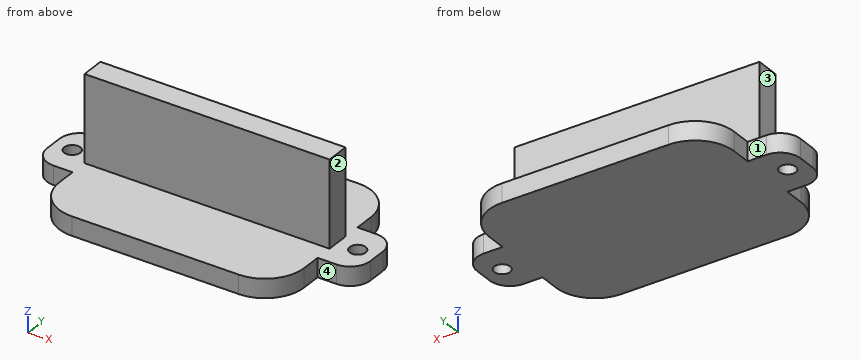
from build123d import *

# Parameters (mm, degrees)
CROQUIS1_R              = 0.85
SALIENTE_EXTRUIR1_DEPTH = 2
CROQUIS2_W              = 26
CROQUIS2_H              = 2.5032448
SALIENTE_EXTRUIR3_DEPTH = 11.15


with BuildPart() as part:
    # Croquis1 → Saliente-Extruir1 (new body)
    # profile 1 of 3: a face of its own
    with BuildSketch(Plane.XY):
        with BuildLine():
            Line((8.85, -9.375), (-8.85, -9.375))
            ThreePointArc((-8.85, -9.375), (-11.784493142, -8.159493142), (-13, -5.225))
            Line((-13, -5.225), (-13, 5.225))
            ThreePointArc((-13, 5.225), (-11.784493142, 8.159493142), (-8.85, 9.375))
            Line((-8.85, 9.375), (8.85, 9.375))
            ThreePointArc((8.85, 9.375), (11.784493142, 8.159493142), (13, 5.225))
            Line((13, 5.225), (13, -5.225))
            ThreePointArc((13, -5.225), (11.784493142, -8.159493142), (8.85, -9.375))
        make_face()
    # profile 2 of 3: a face of its own
    with BuildSketch(Plane.XY):
        with BuildLine():
            Line((-15, -3.125), (-13, -3.125))
            Line((-13, -3.125), (-13, 3.125))
            Line((-13, 3.125), (-15, 3.125))
            ThreePointArc((-15, 3.125), (-16.52027958, 2.49527958), (-17.15, 0.975))
            Line((-17.15, 0.975), (-17.15, -0.975))
            ThreePointArc((-17.15, -0.975), (-16.52027958, -2.49527958), (-15, -3.125))
        make_face()
        with Locations((-15.15, 0)):
            Circle(CROQUIS1_R, mode=Mode.SUBTRACT)
    # profile 3 of 3: a face of its own
    with BuildSketch(Plane.XY):
        with BuildLine():
            Line((13, 3.125), (13, -3.125))
            Line((13, -3.125), (15, -3.125))
            ThreePointArc((15, -3.125), (16.52027958, -2.49527958), (17.15, -0.975))
            Line((17.15, -0.975), (17.15, 0.975))
            ThreePointArc((17.15, 0.975), (16.52027958, 2.49527958), (15, 3.125))
            Line((15, 3.125), (13, 3.125))
        make_face()
        with Locations((15.15, 0)):
            Circle(CROQUIS1_R, mode=Mode.SUBTRACT)
    extrude(amount=SALIENTE_EXTRUIR1_DEPTH)

    # Croquis2 → Saliente-Extruir3 (add)
    with BuildSketch(Plane.XY):
        Rectangle(CROQUIS2_W, CROQUIS2_H)
    extrude(amount=SALIENTE_EXTRUIR3_DEPTH)


solid = part.part
Work out the finished part from the listing and answer in its coordinate system (mm). Face numbers are marked on the shaded views. A direction names the side the tool comes from. Give positions to 0.01 mm unless a question says otherwise; leave off trailing zeros. Order: outer loops, then holes, each group sorted by start corner. A loop starts at its lowest first (then second) coordinate and runs counter-clockwise, first axis right, second up. Notation, with made-up numbers: M 13.5,12.5 L 44.5,12.5 A16 ccw 44.5,42.5 Z; hole C -37.5,52.5 d4. An arc over 180 degrees is marked long. Return JSON: item names as keys, results as strings.
Q1. Each of these flat-tipped pins is pushed along its axis until it touches: pin 1 (1.6 mm diameter, centred on y = -3.5, z = 1, fed in from +X); pin 2 (3 mm diameter, centred on y = -1.5, z = 7.5, fed in from +X); pin 3 (1 mm diameter, centred on x = 15.15, y = 0, fed in from -Z); pin 4 (0.6 mm diameter, centred on y = 4.5, z = 1, fed in from -X). Where does it stop, or does it pass through?
Answer below:
{"pin 1": "stops at x = 16.28", "pin 2": "stops at x = 13", "pin 3": "passes through", "pin 4": "stops at x = -13"}
Q2. Find section B-B, the plane z = 1. Write down the section's boundary in (x, y) (3 decimals), and give its area (3 significant figures).
Answer below:
{"outline": "M -17.15,-0.975 A2.15 ccw -15,-3.125 L -13,-3.125 L -13,-5.225 A4.15 ccw -8.85,-9.375 L 8.85,-9.375 A4.15 ccw 13,-5.225 L 13,-3.125 L 15,-3.125 A2.15 ccw 17.15,-0.975 L 17.15,0.975 A2.15 ccw 15,3.125 L 13,3.125 L 13,5.225 A4.15 ccw 8.85,9.375 L -8.85,9.375 A4.15 ccw -13,5.225 L -13,3.125 L -15,3.125 A2.15 ccw -17.15,0.975 Z; hole C -15.15,0 d1.7; hole C 15.15,0 d1.7", "area": "516 mm^2"}
Q3. Find section A-A, the plane y = 0. Write down the section's boundary in (x, z).
Answer below:
{"outline": "M -17.15,0 L -16,0 L -16,2 L -17.15,2 Z; M -14.3,0 L 14.3,0 L 14.3,2 L 13,2 L 13,11.15 L -13,11.15 L -13,2 L -14.3,2 Z; M 16,0 L 17.15,0 L 17.15,2 L 16,2 Z"}
Q4. Find the intervals of material crossed by line 1 along Y through (x, z) = (-15.15, 0.85); line 2 along Z through (x, y) = (7.5, -4.5); line 3 along Y through (x, z) = (1, 9.75), in increasing order. Write a range as [from, to].
Answer below:
{"line 1": "y = [-3.12, -0.85], [0.85, 3.12]", "line 2": "z = [0, 2]", "line 3": "y = [-1.25, 1.25]"}
Q5. Find section C-C, the plane x = 3. Write down the section's boundary in (y, z) (3 decimals).
Answer below:
{"outline": "M -9.375,0 L 9.375,0 L 9.375,2 L 1.252,2 L 1.252,11.15 L -1.252,11.15 L -1.252,2 L -9.375,2 Z"}
Q6. Find section D-D, the plane z = 8. Write down the section's boundary in (x, y).
Answer below:
{"outline": "M -13,-1.25 L 13,-1.25 L 13,1.25 L -13,1.25 Z"}
Q7. Which of the six approach directions +Z, -Z, +X, -X, +Y, -Y give full straight-line access (tool end or side, diameter ignored) to the marked faces 1, 2, 3 and 4?
Answer below:
{"face 1": "+Z, -Z, -X, +Y", "face 2": "+Z, +X, +Y, -Y", "face 3": "+Z, -X, +Y, -Y", "face 4": "+Z, -Z, +X, -Y"}
